Autodesk Inventor part; units mm, degrees
ref_plane "YZ Plane" through (0, 0, 0) normal (1, 0, 0) x (0, 1, 0)
ref_plane "XZ Plane" through (0, 0, 0) normal (0, 1, 0) x (-1, 0, 0)
ref_plane "XY Plane" through (0, 0, 0) normal (0, 0, 1) x (1, 0, 0)
sketch "Sketch1" plane through (0, 0, 0) normal (0, 1, 0) x (-1, 0, 0)
  line L0 (57.5, -190) -> (57.5, -190) construction
  line L1 (-57.5, -190) -> (-57.5, 0) construction
  line L2 (-57.5, 0) -> (57.5, 0)
  line L3 (57.5, 0) -> (57.5, -190) construction
  line L4 (80.5, 0) -> (-80.5, 0) construction
  line L5 (0, -228) -> (0, 38) construction
  line L6 (57.5, -190) -> (-57.5, -190)
  line L7 (-57.5, -190) -> (-57.5, -190) construction
  line L8 (57.5, 0) -> (-55.1767, 0)
  line L9 (57.5, -40) -> (-57.5, -40) construction
  line L10 (-57.5, -40) -> (-57.5, 0)
  line L11 (-57.5, 0) -> (57.5, 0)
  line L12 (57.5, 0) -> (57.5, -40)
  line L13 (-57.5, -190) -> (-57.5, -40)
  line L14 (57.5, -190) -> (57.5, -40)
  point P0 (0, 0)
  dimension "width" = 115
  dimension "Length" = 190
  dimension "d2" = 115
  dimension "d112" = 40
extrude "Base" add sketch "Sketch1" against normal blind 5
sketch "Sketch11" plane through (0, 0, 0) normal (0, 1, 0) x (1, 0, 0)
  line L0 (0, 228) -> (0, -38) construction
  line L1 (-57.5, 0) -> (57.5, 0) construction
  line L2 (57.5, 190) -> (-57.5, 190)
  line L3 (-50, 5) -> (50, 5) construction
  line L4 (50, 5) -> (50, 35) construction
  line L5 (50, 35) -> (-50, 35) construction
  line L6 (-50, 35) -> (-50, 5) construction
  point P0 (0, 0)
  point P1 (50, 185)
  point P2 (-50, 185)
  dimension "d91" = 5
  dimension "d92" = 50
  dimension "d93" = 5
  dimension "d94" = 50
  dimension "d113" = 30
hole "Mounting Holes" at (50, 0, -5) at (-50, 0, -5) at (50, 0, -185) at (-50, 0, -185) at (-50, 0, -35) at (50, 0, -35) direction (0, -1, 0) diameter 3.4 depth 6
fillet "Fillet1" radius 5 4 edges at (-57.5, -2.5, 0) (57.5, -2.5, -190) (-57.5, -2.5, -190) (57.5, -2.5, 0)
sketch "Sketch12" plane through (0, 0, 0) normal (0, 1, 0) x (1, 0, 0)
  line L0 (-50, 82) -> (-1, 82) construction
  line L1 (-1, 82) -> (-1, 24) construction
  line L2 (-1, 24) -> (-50, 24) construction
  line L3 (-50, 24) -> (-50, 82) construction
  line L4 (-57.5, 185) -> (-57.5, 5)
  line L5 (0, 228) -> (0, -38)
  line L6 (-52.5, 0) -> (52.5, 0)
  circle A0 centre (-50, 35) radius 1.7
  point P0 (0, 0)
  point P1 (0, 0)
  point P2 (52.2987, 0)
  point P3 (-57.5, 40)
  point P4 (0, 0)
  dimension "d103" = 49
  dimension "d104" = 58
  dimension "d239" = 24
hole "RasPi Mounting Holes" at (-50, 0, -82) at (-1, 0, -82) at (-1, 0, -24) at (-50, 0, -24) direction (0, -1, 0) diameter 3.4 depth 6
sketch "Sketch15" plane through (0, 0, 0) normal (0, 1, 0) x (1, 0, 0)
  line L0 (50, 82) -> (50, 20.5) construction
  line L1 (50, 20.5) -> (18, 20.5) construction
  line L2 (18, 20.5) -> (18, 82) construction
  line L3 (18, 82) -> (50, 82) construction
  line L4 (-52.5, 0) -> (52.5, 0)
  circle A0 centre (-1, 82) radius 1.7
  circle A1 centre (50, 35) radius 1.7
  point P0 (0, 0)
  point P1 (0, 0)
  dimension "d122" = 32
  dimension "d123" = 61.5
hole "LM2596 Mounting Holes" at (50, 0, -82) at (50, 0, -20.5) at (18, 0, -20.5) at (18, 0, -82) direction (0, -1, 0) diameter 3.4 depth 6
sketch "Sketch16" plane through (0, 0, 0) normal (0, 1, 0) x (1, 0, 0)
  line L0 (-7.5, 165) -> (7.5, 165) construction
  line L1 (7.5, 165) -> (7.5, 178.5) construction
  line L2 (7.5, 178.5) -> (-7.5, 178.5) construction
  line L3 (-7.5, 178.5) -> (-7.5, 165) construction
  line L4 (52.5, 190) -> (-52.5, 190)
  point P0 (0, 0)
  point P1 (0, 178.5)
  point P2 (0, 190)
  dimension "d132" = 15
  dimension "d133" = 13.5
  dimension "d251" = 11.5
hole "Camera Mount Mounting Holes" at (-7.5, 0, -178.5) at (-7.5, 0, -165) at (7.5, 0, -165) at (7.5, 0, -178.5) direction (0, -1, 0) diameter 3.4 depth 6
sketch "Sketch17" plane through (0, 0, 0) normal (0, 1, 0) x (1, 0, 0)
  line L0 (-57.1973, 19.3379) -> (-57.1973, 79.4802) construction
  line L1 (-57.1973, 79.4802) -> (-14.6793, 79.4802) construction
  line L2 (-14.6793, 79.4802) -> (-14.6793, 19.3379) construction
  line L3 (-14.6793, 19.3379) -> (-57.1973, 19.3379) construction
  circle A0 centre (-50, 24) radius 1.7
  circle A1 centre (-50, 82) radius 1.7
  line L4 (-52.5, 0) -> (52.5, 0)
  spline S0 degree 4 poles (-24.5389, 124.9198) (-24.922, 125.4965) (-27.6826, 126.8954) (-30.1628, 126.7912) (-32.1332, 125.7629) (-33.4299, 124.0907) (-33.6545, 122.2258) (-32.7478, 119.1755) (-29.7631, 118.647) (-24.9617, 117.5574) (-28.1153, 114.1457) (-30.627, 115.8823) (-32.3688, 117.1404) knots 0 0 0 0 0 0.20272 0.281354 0.3552 0.433005 0.51958 0.610323 0.697239 0.780233 1 1 1 1 1
  line L5 (-32.3688, 117.1404) -> (-33.9542, 115.1175)
  line L6 (-24.5389, 124.9198) -> (-25.9227, 122.7407)
  spline S1 degree 4 poles (-25.9227, 122.7407) (-26.5371, 123.0059) (-27.0432, 123.8303) (-29.8104, 124.5696) (-31.1048, 122.982) (-30.4927, 121.5853) (-28.2889, 121.2516) (-27.5721, 120.9152) (-25.6358, 120.2756) (-24.5434, 118.9786) (-23.9735, 117.8945) (-24.2985, 114.6128) (-27.371, 112.453) (-32.008, 112.9595) (-33.5375, 114.8946) (-33.9542, 115.1175) knots 0 0 0 0 0 0.144957 0.205265 0.266901 0.324627 0.385746 0.449034 0.509011 0.57578 0.647336 0.72838 0.816759 1 1 1 1 1
  line L7 (-23.2822, 126.3237) -> (-23.2822, 113.2811)
  line L8 (-23.2822, 113.2811) -> (-20.5533, 113.2884)
  line L9 (-20.5533, 113.2884) -> (-20.5533, 117.1404)
  line L10 (-20.5436, 123.784) -> (-20.5436, 119.7226)
  line L11 (-20.5436, 119.7226) -> (-18.2264, 119.7226)
  line L12 (-20.5436, 123.784) -> (-18.2264, 123.784)
  line L13 (-23.2822, 126.3237) -> (-18.1485, 126.3237)
  line L14 (-20.5533, 117.1404) -> (-18.1485, 117.1404)
  spline S2 degree 4 poles (-18.1485, 126.3237) (-16.6845, 126.5227) (-13.988, 125.7234) (-13.1568, 120.9814) (-14.2131, 118.7079) (-16.0401, 117.1114) (-18.1485, 117.1404) knots 0 0 0 0 0 0.42308 0.582818 1 1 1 1 1
  spline S3 degree 4 poles (-18.2264, 123.784) (-16.7633, 123.9916) (-15.1954, 121.9939) (-16.394, 119.8116) (-18.2264, 119.7226) knots 0 0 0 0 0 1 1 1 1 1
  line L15 (-9.8541, 122.5443) -> (-9.8541, 113.2671)
  line L16 (-9.8541, 113.2671) -> (-6.5382, 113.2671)
  line L17 (-6.5382, 113.2671) -> (-6.5382, 113.4426)
  line L18 (-6.5382, 113.4426) -> (-6.5382, 117.1888)
  line L19 (-6.5382, 117.1888) -> (-4.8269, 117.1888)
  line L20 (-4.8269, 117.1888) -> (-2.3071, 113.2671)
  line L21 (-2.3071, 113.2671) -> (1.6946, 113.2671)
  line L22 (1.6946, 113.2671) -> (-0.8253, 117.1888)
  line L23 (-9.8541, 122.5443) -> (-6.5382, 122.5443)
  line L24 (-6.5382, 122.5443) -> (-6.5382, 120.5743)
  line L25 (-6.5382, 120.5743) -> (-2.6026, 120.5743)
  line L26 (-2.6026, 120.5743) -> (-2.6026, 123.1634)
  line L27 (-2.6026, 123.1634) -> (-9.8541, 123.1634)
  line L28 (-9.8541, 123.1634) -> (-9.8541, 126.4713)
  line L29 (-9.8541, 126.4713) -> (-0.5373, 126.4713)
  line L30 (0.769, 125.022) -> (0.769, 118.8518)
  arc A2 (-0.8253, 117.1888) -> (0.769, 118.8518) centre (-0.9621, 118.9157) ccw
  arc A3 (0.769, 125.022) -> (-0.5373, 126.4713) centre (-1.5712, 124.2261) ccw
  line L31 (2.6608, 126.4713) -> (6.0256, 126.4713)
  line L32 (6.0256, 126.4713) -> (6.0256, 113.2671)
  line L33 (6.0256, 113.2671) -> (2.6608, 113.2671)
  line L34 (2.6608, 113.2671) -> (2.6608, 126.4713)
  line L35 (7.5596, 126.4713) -> (7.5596, 123.1634)
  line L36 (7.5596, 123.1634) -> (10.9283, 123.1634)
  line L37 (10.9283, 123.1634) -> (10.9283, 113.2671)
  line L38 (10.9283, 113.2671) -> (14.2393, 113.2671)
  line L39 (14.2393, 113.2671) -> (14.2393, 126.4713)
  line L40 (14.2393, 126.4713) -> (7.5596, 126.4713)
  line L41 (14.8531, 126.4713) -> (14.8531, 123.1634)
  line L42 (14.8531, 123.1634) -> (17.2975, 123.1634)
  line L43 (17.2975, 123.1634) -> (19.544, 126.4713)
  line L44 (19.544, 126.4713) -> (14.8531, 126.4713)
  line L45 (20.2187, 126.4775) -> (20.2187, 113.2671)
  line L46 (20.2187, 113.2671) -> (23.5406, 113.2671)
  line L47 (23.5406, 113.2671) -> (23.5406, 126.4775)
  line L48 (23.5406, 126.4775) -> (20.2187, 126.4775)
  line L49 (24.1159, 121.5593) -> (24.1159, 118.2075)
  line L50 (24.1159, 118.2075) -> (26.608, 118.2075)
  line L51 (26.608, 118.2075) -> (26.608, 121.5593)
  line L52 (26.608, 121.5593) -> (24.1159, 121.5593)
  line L53 (23.5406, 126.4775) -> (23.5406, 123.1396)
  line L54 (23.5406, 123.1396) -> (28.6492, 123.1396)
  line L55 (28.6492, 123.1396) -> (28.6492, 126.4775)
  line L56 (28.6492, 126.4775) -> (23.5406, 126.4775)
  line L57 (28.6492, 126.4775) -> (30.8175, 123.1396)
  line L58 (30.8175, 123.1396) -> (28.6492, 123.1396)
  line L59 (26.608, 121.5593) -> (28.8205, 121.5315)
  line L60 (28.8205, 121.5315) -> (26.608, 118.2075)
  line L61 (23.5406, 116.6064) -> (30.8177, 116.6064)
  line L62 (30.8177, 116.6064) -> (28.6492, 113.2671)
  line L63 (28.6492, 113.2671) -> (23.5406, 113.2671)
  line L64 (-20.5533, 113.2884) -> (-7.3915, 113.2884)
  line L65 (-57.5, 185) -> (-57.5, 5)
  line L66 (57.5, 5) -> (57.5, 185)
  line L67 (57.5, 185) -> (57.5, 5)
  point P0 (0, 0)
  point P1 (-35.9383, 19.3379)
  point P2 (0, 0)
  point P3 (-26.0743, 125.9223)
  point P4 (-28.9193, 126.6257)
  point P5 (-32.067, 125.6116)
  point P6 (-33.4554, 122.3675)
  point P7 (-29.2911, 118.5075)
  point P8 (-26.9401, 117.3059)
  point P9 (-27.1681, 116.1283)
  point P10 (-28.939, 115.4933)
  point P11 (-32.4456, 119.8309)
  point P12 (-33.1379, 124.2152)
  point P13 (-30.7742, 126.3572)
  point P14 (-26.7112, 123.2461)
  point P15 (-28.1768, 123.919)
  point P16 (-30.0893, 123.8265)
  point P17 (-30.7803, 122.924)
  point P18 (-30.2965, 121.8845)
  point P19 (-28.5195, 121.2364)
  point P20 (-27.4225, 120.886)
  point P21 (-25.8005, 120.143)
  point P22 (-24.69, 119.0688)
  point P23 (-24.2101, 117.9282)
  point P24 (-24.53, 115.3475)
  point P25 (-26.7119, 113.3702)
  point P26 (-30.6972, 113.2718)
  point P27 (-33.2613, 114.5685)
  point P28 (-15.6674, 125.8448)
  point P29 (-14.0095, 123.9105)
  point P30 (-13.6514, 121.4185)
  point P31 (-14.0618, 119.634)
  point P32 (-15.2337, 118.127)
  point P33 (-16.9529, 123.3565)
  point P34 (-16.2765, 122.0378)
  point P35 (-16.6728, 120.5472)
  point P36 (0, 106.588)
extrude "SP RITE" cut sketch "Sketch17" against normal blind 2 contours L6 S1 L5 S0 | L13 S2 L14 L9 L8 L7 | L15 L23 L24 L25 L26 L27 L28 L29 A3 L30 A2 L22 L21 L20 L19 L18 L17 L16 | L12 S3 L11 L10 | L31 L32 L33 L34 | L40 L39 L38 L37 L36 L35 | L44 L43 L42 L41 | L48 L47 L46 L45 | L56 L55 L54 L47 | L47 L61 L62 L63 | L57 L58 L55 | L52 L51 L50 L49 | L59 L60 L51
equation "\"d2\" = width"
equation "\"d95\" = HoleDia"
equation "\"d105\" = HoleDia"
equation "\"d125\" = HoleDia"
equation "\"d135\" = HoleDia"
equation "\"HoleDia\" = 3.4"
properties part number "top plate"
Read the model definition and answer for the solid it produces. Units are mm, in the model's axes. A direction names the side the tool comes from. Round coordinates to 2 decimals unless told otherwise and drop trailing zeros. Use CSV: the item, a comma, the result in double quotes.
Q1. Determine the mould class of faces 1 (the flat face through (-1, -2, -190)), 2 (the flat face through (26, -2, -120)) for opening direction Z: +Z half, -Z half, draft (parallel to the pull), parting line (faces both ways), or undercut.
Values:
face 1,"-Z half"
face 2,"undercut"
Q2. Straight lines are drawn through the part: line 1 along Z through (x, y) = (7.5, -3.6); line 2 along Z through (x, y) = (-1, -3.4); line 3 along X through (y, z) = (-1.35, -82). For each, find the intervals that lie inside material, in ascending order.
Values:
line 1,"z = -190 to -180.2, -176.8 to -166.7, -163.3 to 0"
line 2,"z = -190 to -83.7, -80.3 to -25.7, -22.3 to 0"
line 3,"x = -57.5 to -51.7, -48.3 to -2.7, 0.7 to 16.3, 19.7 to 48.3, 51.7 to 57.5"
Q3. This flat-tipped pin is pushed along its axis until it touches: pin 1 Ø2.5 at (x, z) = (18, -20.5) entering from -Y. Where does it stop, or does it pass through?
Values:
pin 1,"passes through"
Q4. Find section A-A, the plane y = -1. Count the separate pieces of the cut face and the enclosed holes in it, then the cut area to 3 significant figures.
Values:
separate pieces,"1"
enclosed holes,"26"
area,"21,200 mm²"
Q5. A tool of negligible diameter and unlimited length cuts with its end or side. For faces 3 (the flat face through (-29, -2, -120)), 4 (the cylindrical face through (-1.07, -2.54, -83.7)), from which of +Z, -Z, +X, -X, +Y, -Y can it reach the whole face along a straight path? Write none if from no direction.
Values:
face 3,"+Y"
face 4,"+Y, -Y"
